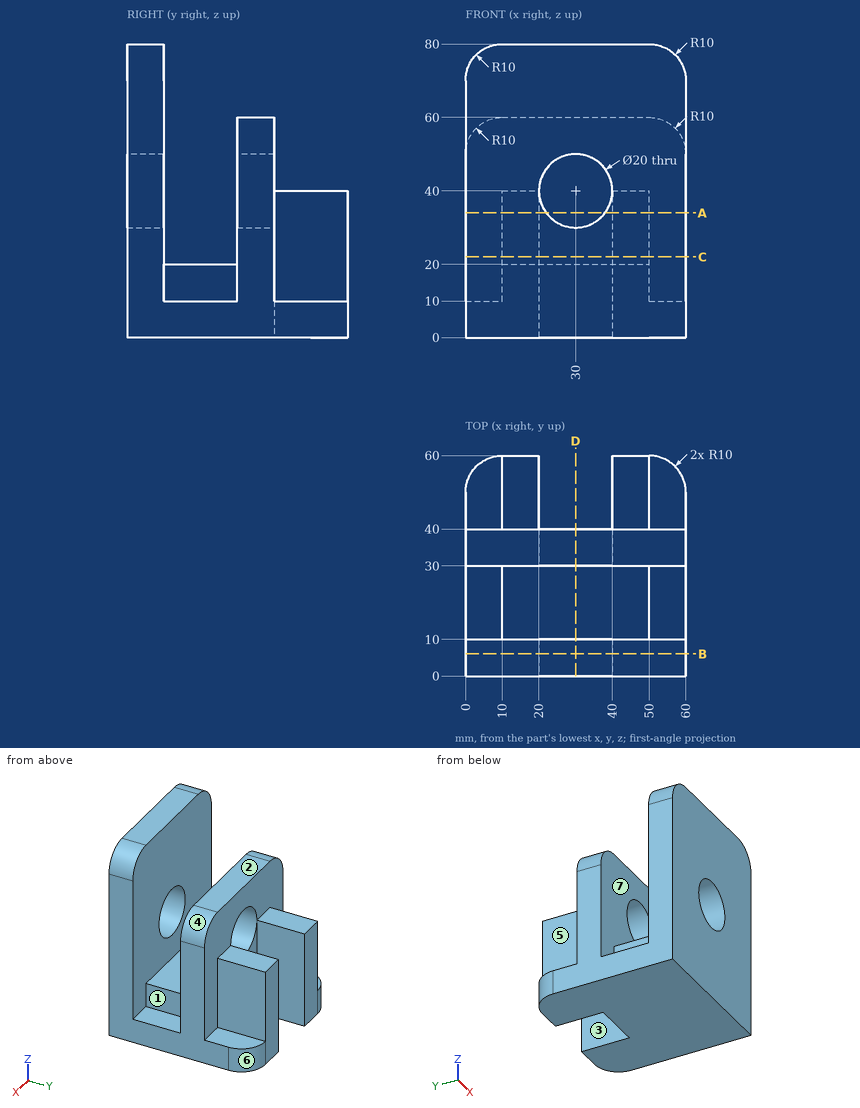
For this review, use the dimensioned drawing (mm, ordinates from the lowest corner) and the shaded views. A direction names the side the tool comes from. Round coordinates to 2 decimals unless told otherwise and drop trailing zeros. Write each loop counter-clockwise with the first axis right and the second up, starting at its lowest first coordinate (ties: lowest second). Pieces come first, ordered by that corner, then holes. Notation, with made-up numbers: (64, -12) -> (93, -12) arc R12 ccw to (93, -1) -> close; hole circle Ø8 at (33.25, -27.75). An arc over 180 degrees is marked (long way). Use CSV: the item, a comma, the result in double quotes.
Q1. Consider section A-A (z = 34). Give the boundary of the cut face in (x, y).
Checks:
outline,"(0, 0) -> (22, 0) -> (22, 10) -> (0, 10) -> close; (0, 30) -> (22, 30) -> (22, 40) -> (20, 40) -> (20, 60) -> (10, 60) -> (10, 40) -> (0, 40) -> close; (38, 0) -> (60, 0) -> (60, 10) -> (38, 10) -> close; (38, 30) -> (60, 30) -> (60, 40) -> (50, 40) -> (50, 60) -> (40, 60) -> (40, 40) -> (38, 40) -> close"
Q2. Mouldability with a two-part tool opening along Y and no side actions: class the marked faces 5, 6 and 7 as released by +Y, released by -Y, zero draft, split by the parting line, or undercut.
Checks:
face 5,"zero draft"
face 6,"released by +Y"
face 7,"undercut"
Q3. For pin 1 Ø3 at (x, y) = (14.5, 47) entering from +Z; pin 2 Ø6 at (x, z) = (32, 23) entering from +Y; pin 3 Ø12 at (y, z) = (25, 69) entering from -X; pin 4 Ø16 at (y, z) = (54, 30) entering from -X, all flat-tipped, find the tip position at first contact; note any pin that passes through.
Checks:
pin 1,"z = 40"
pin 2,"y = 40"
pin 3,"through"
pin 4,"x = 10"
Q4. For the marked faces 1, 2, 3 and 4, list the 3-axis set-ups (+Z, -Z, +X, -X, +Y, -Y) from which the entire face can be reached by the end or side of a thin tool; tool diameter is ignored.
Checks:
face 1,"+Z, +X"
face 2,"+Z, +X, -X, +Y"
face 3,"+Z, -Z, +Y"
face 4,"+Z, +X, +Y"
Q5. Consider section B-B (y = 6). Give the boundary of the cut face in (x, z), then the cut area to 3 significant figures.
Checks:
outline,"(0, 0) -> (60, 0) -> (60, 70) arc R10 ccw to (50, 80) -> (10, 80) arc R10 ccw to (0, 70) -> close; hole circle Ø20 at (30, 40)"
area,"4,440 mm²"
Q6. Consider section D-D (x = 30). Give the boundary of the cut face in (y, z).
Checks:
outline,"(0, 0) -> (40, 0) -> (40, 30) -> (30, 30) -> (30, 20) -> (10, 20) -> (10, 30) -> (0, 30) -> close; (0, 50) -> (10, 50) -> (10, 80) -> (0, 80) -> close; (30, 50) -> (40, 50) -> (40, 60) -> (30, 60) -> close"
Q7. To check wall thickness, follow probe 1 along X at (y, z) = (3.25, 40); probe 2 along Y at (x, z) = (8, 55.5); probe 3 along X at (y, z) = (43, 35). State the ranges of each line that lie inside material, in increasing order. Write a range as [from, to].
Checks:
probe 1,"[0, 20], [40, 60]"
probe 2,"[0, 10], [30, 40]"
probe 3,"[10, 20], [40, 50]"
Q8. Consider section C-C (z = 22). Give the boundary of the cut face in (x, y).
Checks:
outline,"(0, 0) -> (60, 0) -> (60, 10) -> (0, 10) -> close; (0, 30) -> (60, 30) -> (60, 40) -> (50, 40) -> (50, 60) -> (40, 60) -> (40, 40) -> (20, 40) -> (20, 60) -> (10, 60) -> (10, 40) -> (0, 40) -> close"
